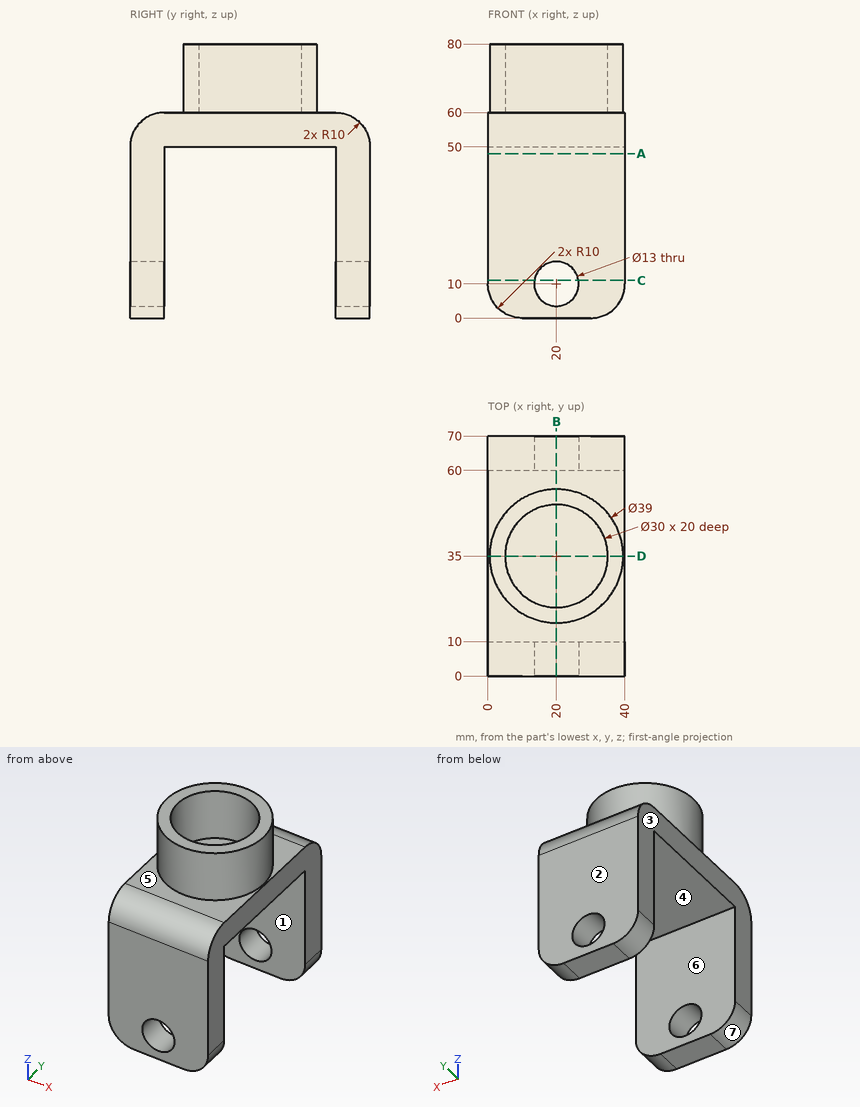
Geometry check sheet. Reference: drawing and pictorial views, mm from the part's lowest x, y, z. A direction names the side the tool comes from. Give positions to 0.01 mm unless a question says otherwise; leave off trailing zeros. Loops run counter-clockwise (first coordinate to the right, second up) from the corner with the lowest first, then second, coordinate; pieces in that order, holes last.
1. Thickness scan on line 1 (Y direction, x = 35, z = 7.5); line 2 (Y direction, x = 20, z = 70); line 3 (X direction, y = 7.5, z = 10). Record the ranges inside material, lowest first.
2. Section check B-B, the plane x = 20. Enter the section's corners in (y, z), then the cut area to 3 significant figures.
3. Section check C-C, the plane z = 11. Enter the section's corners in (x, y).
4. Go/stop test with flat-tipped pins: pin 1 Ø11.5 at (x, z) = (20, 10) entering from -Y; pin 2 Ø1.5 at (x, z) = (4.5, 70.5) entering from +Y; pin 3 Ø1.5 at (x, y) = (19.5, 41) entering from -Z; pin 4 Ø10 at (x, y) = (9, 60.5) entering from +Z. Record where each tip stops, or that it passes through.
5. Set-up check for the marked faces 5, 6 and 7: record each of +Z, -Z, +X, -X, +Y, -Y from which the full face is reachable in a straight line by a thin tool's end or side.
6. Mould release check, pull along Y, two halves, no side actions. Record for the marked faces 1, 2, 3 and 4: released by +Y, released by -Y, zero draft, split by the parting line, or undercut.
7. Section check D-D, the plane y = 35. Enter the section's corners in (x, z).
8. Section check A-A, the plane z = 48. Enter the section's corners in (x, y).
Geometry says:
1. line 1: y = 0 to 10, 60 to 70
1. line 2: y = 15.5 to 20, 50 to 54.5
1. line 3: x = 0 to 13.5, 26.5 to 40
2. outline: (0, 0) - (10, 0) - (10, 3.5) - (0, 3.5) - close; (0, 16.5) - (10, 16.5) - (10, 50) - (60, 50) - (60, 16.5) - (70, 16.5) - (70, 50) arc R10 ccw to (60, 60) - (54.5, 60) - (54.5, 80) - (50, 80) - (50, 60) - (20, 60) - (20, 80) - (15.5, 80) - (15.5, 60) - (10, 60) arc R10 ccw to (0, 50) - close; (60, 0) - (70, 0) - (70, 3.5) - (60, 3.5) - close
2. area: 1,580 mm2
3. outline: (0, 0) - (13.58, 0) - (13.58, 10) - (0, 10) - close; (0, 60) - (13.58, 60) - (13.58, 70) - (0, 70) - close; (26.42, 0) - (40, 0) - (40, 10) - (26.42, 10) - close; (26.42, 60) - (40, 60) - (40, 70) - (26.42, 70) - close
4. pin 1: passes through
4. pin 2: stops at y = 47.75
4. pin 3: stops at z = 50
4. pin 4: stops at z = 60
5. face 5: +Z
5. face 6: -Z, +X, -X
5. face 7: -Z, -X, +Y, -Y
6. face 1: undercut
6. face 2: released by +Y
6. face 3: zero draft
6. face 4: undercut
7. outline: (0, 50) - (40, 50) - (40, 60) - (39.5, 60) - (39.5, 80) - (35, 80) - (35, 60) - (5, 60) - (5, 80) - (0.5, 80) - (0.5, 60) - (0, 60) - close
8. outline: (0, 0) - (40, 0) - (40, 10) - (0, 10) - close; (0, 60) - (40, 60) - (40, 70) - (0, 70) - close
